The drawing under review shows one solid part. Ordinate dimensions are in mm from its lowest x, y, z. A direction names the side the tool comes from. Give positions to 0.01 mm unless a question says otherwise; leave off trailing zeros. Loops run counter-clockwise (first coordinate to the right, second up) from the corner with the lowest first, then second, coordinate; pieces in that order, holes last. Notation, with made-up numbers: M 74.5,-39 L 110.5,-39 A25 cw 110.5,-7 Z; hole C 84,-17 d5. An arc over 180 degrees is marked long. One line per item, written item: value. Start each with the question number.
Q1. Mouldability with a two-part tool opening along Y and no side actions: class the marked faces 1, 2 and 3 as released by +Y, released by -Y, zero draft, split by the parting line, or undercut.
Q2. For the marked faces 4, 5 and 6, list the 3-axis set-ups (+Z, -Z, +X, -X, +Y, -Y) from which the entire face can be reached by the end or side of a thin tool; tool diameter is ignored.
Q3. We need section D-D on z = 9.5. Write out the cut boundary in (x, y), plus the area to 3 significant figures.
Q4. We need section A-A on y = 12.7. Write out the cut boundary in (x, z) (3 decimals).
Q5. We need section B-B on x = 38.1. Write out the cut boundary in (y, z) (3 decimals).
Q6. We need section C-C on x = 12.7. Write out the cut boundary in (y, z) (3 decimals), plus the area to 3 significant figures.
Q7. For pin 1 (5 mm diameter, centred on x = 54.5, z = 30, fed in from +Y); pin 2 (5 mm diameter, centred on x = 30, y = 44.5, fed in from +Z); pin 3 (10 mm diameter, centred on y = 35, z = 21, fed in from +X); pin 4 (7 mm diameter, centred on x = 12.7, y = 38.1, fed in from +Z) (3 decimals), all flat-tipped, find the tip position at first contact; note any pin that passes through.
Q8. To check wall thickness, follow line 1 along Y through (x, z) = (12.7, 29); line 2 along Y through (x, z) = (12.7, 15); line 3 along Y through (x, z) = (63.5, 30.75). State the ranges of each line that lie inside material, in increasing order. Write a range as from..to.
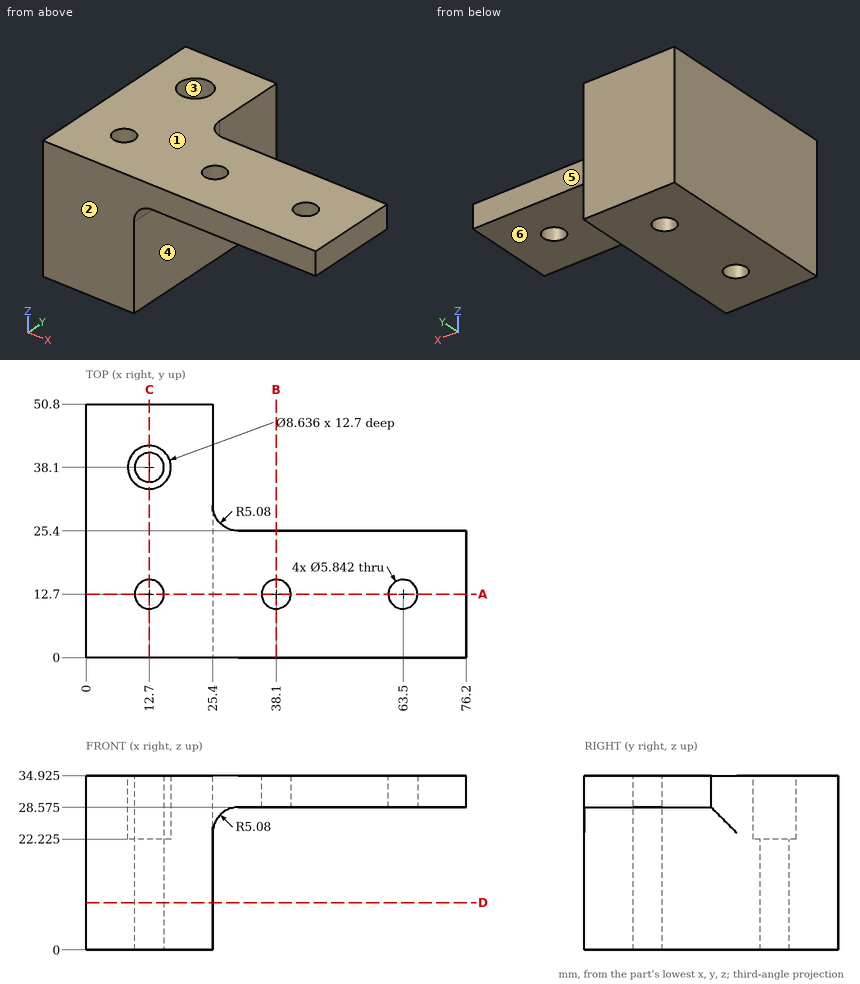
Solved:
1. face 1: zero draft
1. face 2: released by -Y
1. face 3: undercut
2. face 4: -Z, +X, +Y
2. face 5: +Z, -Z, +X, +Y
2. face 6: -Z, +X, +Y, -Y
3. outline: M 0,0 L 25.4,0 L 25.4,50.8 L 0,50.8 Z; hole C 12.7,12.7 d5.84; hole C 12.7,38.1 d5.84
3. area: 1,240 mm2
4. outline: M 0,0 L 9.779,0 L 9.779,34.925 L 0,34.925 Z; M 15.621,0 L 25.4,0 L 25.4,23.495 A5.08 cw 30.48,28.575 L 35.179,28.575 L 35.179,34.925 L 15.621,34.925 Z; M 41.021,28.575 L 60.579,28.575 L 60.579,34.925 L 41.021,34.925 Z; M 66.421,28.575 L 76.2,28.575 L 76.2,34.925 L 66.421,34.925 Z
5. outline: M 0,28.575 L 9.779,28.575 L 9.779,34.925 L 0,34.925 Z; M 15.621,28.575 L 25.4,28.575 L 25.4,34.925 L 15.621,34.925 Z
6. outline: M 0,0 L 9.779,0 L 9.779,34.925 L 0,34.925 Z; M 15.621,0 L 35.179,0 L 35.179,22.225 L 33.782,22.225 L 33.782,34.925 L 15.621,34.925 Z; M 41.021,0 L 50.8,0 L 50.8,34.925 L 42.418,34.925 L 42.418,22.225 L 41.021,22.225 Z
6. area: 1,330 mm2
7. pin 1: y = 25.4
7. pin 2: through
7. pin 3: x = 25.4
7. pin 4: z = 22.225
8. line 1: 0..9.78, 15.62..33.78, 42.42..50.8
8. line 2: 0..9.78, 15.62..35.18, 41.02..50.8
8. line 3: 0..9.78, 15.62..25.4
